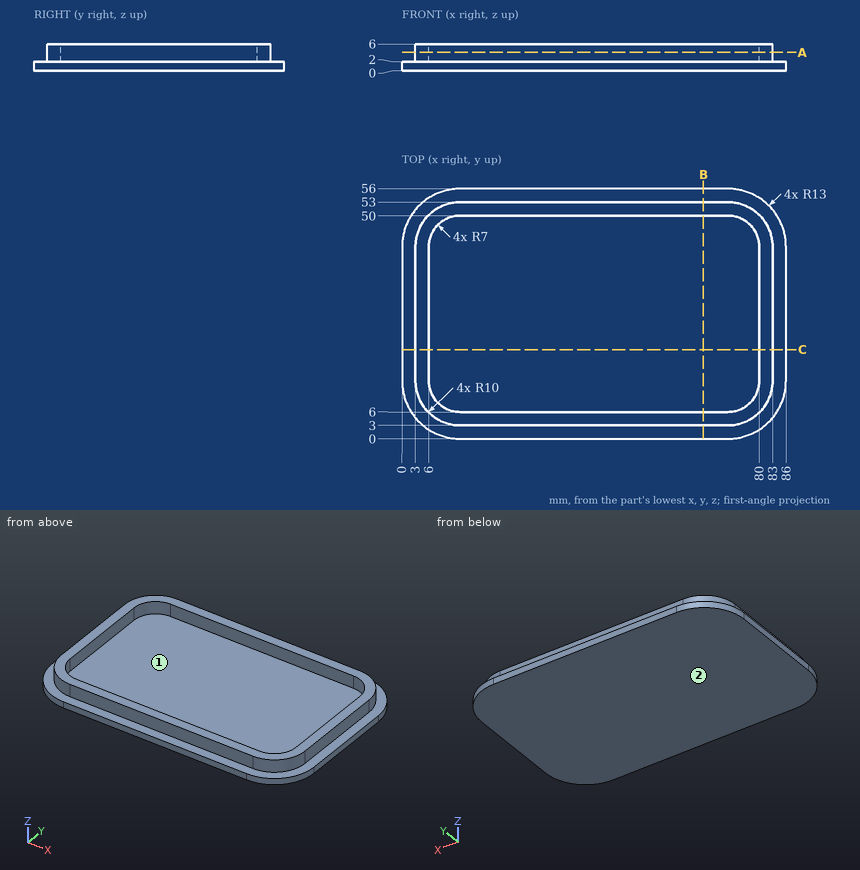
Geometry: see drawing. Coordinates: mm, zero at the bounding-box minimum. Give positions to 0.01 mm unless a question says otherwise; leave off trailing zeros. Loops run counter-clockwise (first coordinate to the right, second up) from the corner with the lowest first, then second, coordinate; pieces in that order, holes last. Notation, with made-up numbers: (-19.75, 62.5) - (36.25, 62.5) arc R25 cw to (36.25, 93.5) - close; hole circle Ø1 at (-23.75, -26). An arc over 180 degrees is marked (long way). Use CSV: the item, a comma, the result in double quotes. Start each with the question number.
1. Draft query along Y for the marked faces 1 and 2. Return one class per face: +Y half, -Y half, draft (parallel to the pull), parting line (faces both ways), or undercut.
2. Section B-B (x = 67.5). Output: boundary loops of the cut face in (y, z).
3. Ray query, L1, parallel to X at y = 15, z = 4; L2, parallel to Y at x = 36, z = 2.4; L3, parallel to Z at x = 75, y = 37.5. Return the intervals inside material, ascending.
4. Pin query (flat end, axial travel): pin 1 (2 mm diameter, centred on y = 36, z = 5.5, fed in from +X); pin 2 (3 mm diameter, centred on x = 52.5, z = 4.5, fed in from -Y); pin 3 (1.2 mm diameter, centred on x = 28.5, z = 4.5, fed in from +Y). Return the tip coordinate at first contact, or that it passes through.
5. Section A-A (z = 4.15). Output: boundary loops of the cut face in (x, y), then the cut area to 3 significant figures.
6. Section C-C (y = 20). Output: boundary loops of the cut face in (x, z), then the cut area to 3 significant figures.
Response:
1,face 1,"undercut"
1,face 2,"draft"
2,outline,"(0, 0) - (56, 0) - (56, 2) - (53, 2) - (53, 6) - (50, 6) - (50, 2) - (6, 2) - (6, 6) - (3, 6) - (3, 2) - (0, 2) - close"
3,L1,"3 to 6, 80 to 83"
3,L2,"3 to 6, 50 to 53"
3,L3,"0 to 2"
4,pin 1,"x = 83"
4,pin 2,"y = 3"
4,pin 3,"y = 53"
5,outline,"(3, 13) arc R10 ccw to (13, 3) - (73, 3) arc R10 ccw to (83, 13) - (83, 43) arc R10 ccw to (73, 53) - (13, 53) arc R10 ccw to (3, 43) - close; hole (6, 13) arc R7 ccw to (13, 6) - (73, 6) arc R7 ccw to (80, 13) - (80, 43) arc R7 ccw to (73, 50) - (13, 50) arc R7 ccw to (6, 43) - close"
5,area,"700 mm²"
6,outline,"(0, 0) - (86, 0) - (86, 2) - (83, 2) - (83, 6) - (80, 6) - (80, 2) - (6, 2) - (6, 6) - (3, 6) - (3, 2) - (0, 2) - close"
6,area,"196 mm²"
